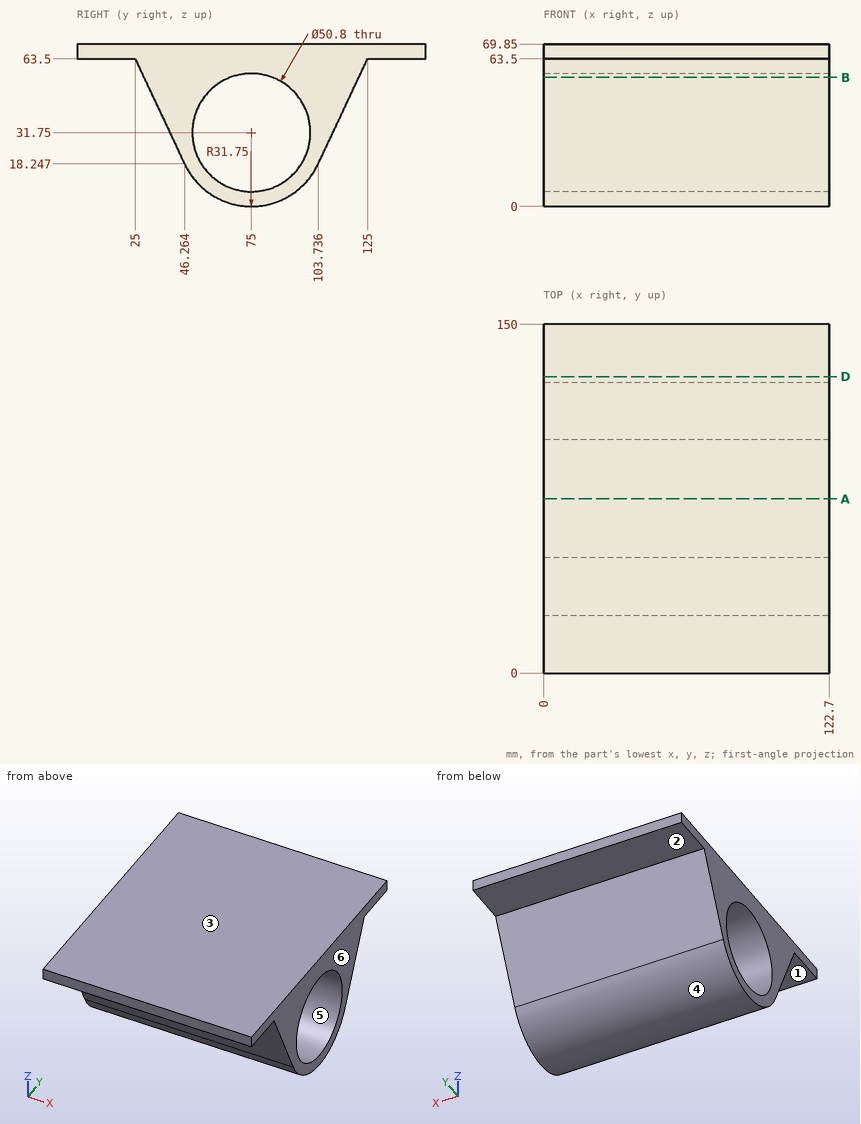
Study the drawing (mm; zero at the part's minimum x, y, z) and answer. A direction names the side the tool comes from. Give positions to 0.01 mm unless a question says otherwise; leave off trailing zeros. Write each loop counter-clockwise with the first axis right and the second up, starting at its lowest first coordinate (ties: lowest second). Pieces come first, ordered by that corner, then holes.
(1) The part is cut by section B-B on z = 55.5. Write down the section's boundary in (x, y) (1 decimal).
Final values:
outline: (0, 28.8) - (122.7, 28.8) - (122.7, 66) - (0, 66) - close; (0, 84) - (122.7, 84) - (122.7, 121.2) - (0, 121.2) - close
(2) Flat-ended cylindrical pins translate along their axes: pin 1 Ø12.5 at (x, y) = (34, 7) entering from -Z; pin 2 Ø2 at (x, z) = (39.5, 34.5) entering from -Y; pin 3 Ø1.5 at (x, y) = (94.5, 66) entering from -Z. Find the tip coordinate at first contact, or state that the pin passes through.
Final values:
pin 1: stops at z = 63.5
pin 2: stops at y = 38.16
pin 3: stops at z = 1.09
(3) The part is cut by section A-A on y = 75. Write down the section's boundary in (x, z), plus the area to 3 significant figures.
Final values:
outline: (0, 0) - (122.7, 0) - (122.7, 6.35) - (0, 6.35) - close; (0, 57.15) - (122.7, 57.15) - (122.7, 69.85) - (0, 69.85) - close
area: 2,340 mm2
(4) Straight lines are drawn through the part: line 1 (Z direction, x = 27, y = 75); line 2 (Z direction, x = 106.5, y = 140.5); line 3 (Y direction, x = 28.5, z = 34.5). For each, find the intervals that lie inside material, in ascending order.
Final values:
line 1: z = 0 to 6.35, 57.15 to 69.85
line 2: z = 63.5 to 69.85
line 3: y = 38.63 to 49.75, 100.25 to 111.37
(5) The part is cut by section D-D on y = 127.5. Write down the section's boundary in (x, z).
Final values:
outline: (0, 63.5) - (122.7, 63.5) - (122.7, 69.85) - (0, 69.85) - close
(6) The mould has two halves that part along Y. Classify the marked faces 4, 5 and 6: pulls with the +Y half, pulls with the -Y half, needs draft (parallel to the pull), parting line crosses it, or undercut.
Final values:
face 4: parting line crosses it
face 5: undercut
face 6: needs draft
(7) Which of the six approach directions +Z, -Z, +X, -X, +Y, -Y give full straight-line access (tool end or side, diameter ignored) to the marked faces 1, 2 and 3?
Final values:
face 1: -Z, +X, -X, -Y
face 2: -Z, +X, -X, +Y
face 3: +Z, +X, -X, +Y, -Y
